```python
from build123d import *

# Parameters (mm, degrees)
SKETCH_1_W          = 100
SKETCH_1_H          = 15
EXTRUDE_1_DEPTH     = 8
SKETCH_2_R          = 2.5
CUT_EXTRUDE_2_DEPTH = 8
FILLET_2_R          = 2.5


with BuildPart() as part:
    # Эскиз1 → Вытянуть1 (new body)
    with BuildSketch(Plane.XY):
        with Locations((50, 7.5)):
            Rectangle(SKETCH_1_W, SKETCH_1_H)
    extrude(amount=EXTRUDE_1_DEPTH)

    # Эскиз2 → Вытянуть2 (cut)
    with BuildSketch(Plane.XY.offset(8)):
        with Locations((5, 7.5)):
            Circle(SKETCH_2_R)
        with BuildLine():
            Line((15, 10), (90, 10))
            ThreePointArc((90, 10), (92.5, 7.5), (90, 5))
            Line((90, 5), (15, 5))
            ThreePointArc((15, 5), (12.5, 7.5), (15, 10))
        make_face()
    extrude(amount=-CUT_EXTRUDE_2_DEPTH, mode=Mode.SUBTRACT)

    # Скругление2
    fillet_2_edges = [part.edges().sort_by_distance(p)[0] for p in [
        (0, 15, 4),
        (100, 15, 4),
        (100, 0, 4),
        (0, 0, 4),
    ]]
    fillet(fillet_2_edges, radius=FILLET_2_R)


solid = part.part
```
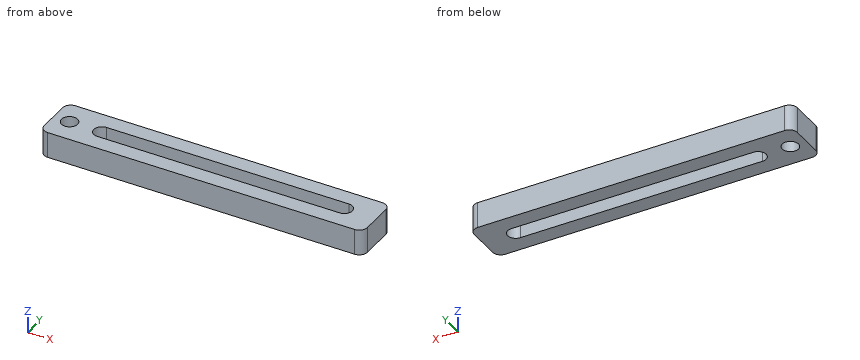
Geometry: final body of the model. Coordinates: model frame, mm. Round coordinates to 2 decimals unless told otherwise and drop trailing zeros. Write each loop counter-clockwise with the first axis right and the second up, starting at its lowest first coordinate (ties: lowest second). Pieces come first, ordered by that corner, then holes.
Item 1: Section query C-C (z = 6.5). Return loops of the section in (x, y).
Item 2: Section query A-A (y = 9). Return loops of the section in (x, z).
Item 3: Material intervals for L1, parallel to Y at x = 61, z = 6; L2, parallel to X at y = 8.25, z = 4.25; L3, parallel to X at y = 5.25, z = 0.5, sorted ascending.
Item 4: Section query B-B (x = 21). Return loops of the section in (y, z).
Completed:
1. outline: (0, 2.5) arc R2.5 ccw to (2.5, 0) - (97.5, 0) arc R2.5 ccw to (100, 2.5) - (100, 12.5) arc R2.5 ccw to (97.5, 15) - (2.5, 15) arc R2.5 ccw to (0, 12.5) - close; hole circle Ø5 at (5, 7.5); hole (15, 5) - (90, 5) arc R2.5 ccw to (90, 10) - (15, 10) arc R2.5 ccw to start
2. outline: (0, 0) - (3, 0) - (3, 8) - (0, 8) - close; (7, 0) - (13, 0) - (13, 8) - (7, 8) - close; (92, 0) - (100, 0) - (100, 8) - (92, 8) - close
3. L1: y = 0 to 5, 10 to 15
3. L2: x = 0 to 2.62, 7.38 to 12.62, 92.38 to 100
3. L3: x = 0 to 3.91, 6.09 to 13.91, 91.09 to 100
4. outline: (0, 0) - (5, 0) - (5, 8) - (0, 8) - close; (10, 0) - (15, 0) - (15, 8) - (10, 8) - close
